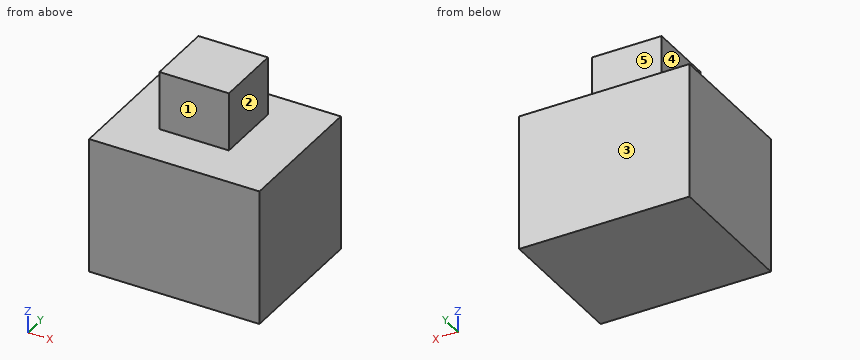
from build123d import *

# Parameters (mm, degrees)
F0_W     = 101.6
F0_H     = 105.0883368849
F1_DEPTH = 101.1590287089
F2_W     = 105.0883368849
F2_H     = 101.1590287089
F3_DEPTH = 25.4
F6_W     = 51.8510639668
F6_H     = 50.3680855036
F7_DEPTH = 43.5765609145


# Not quite as in the source:
# - the program builds the solid bodies; features that only make, move or delete a surface that nothing else refers to are left out


with BuildPart() as f1:
    # F0 (on Top) → F1 (new body)
    with BuildSketch(Plane.XY):
        with Locations((-2.9358975589, -0.3588087857)):
            Rectangle(F0_W, F0_H)
    extrude(amount=F1_DEPTH)

    # F2 (on face) → F3 (join)
    with BuildSketch(Plane.YZ.offset(47.8641024411)):
        with Locations((-0.3588087857, 50.5795143545)):
            Rectangle(F2_W, F2_H)
    extrude(amount=F3_DEPTH)

    # F6 (on face) → F7 (join)
    with BuildSketch(Plane.XY.offset(101.1590287089)):
        with Locations((5.4090619087, 5.453877151)):
            Rectangle(F6_W, F6_H)
    extrude(amount=F7_DEPTH)


solid = f1.part
Geometry: final body of the model. Coordinates: model frame, mm. Face numbers are marked on the shaded views. A direction names the side the tool comes from. Give positions to 0.01 mm unless a question says otherwise; leave off trailing zeros. Write each loop counter-clockwise with the first axis right and the second up, starting at its lowest first coordinate (ties: lowest second). Pieces come first, ordered by that corner, then holes. Notation, with made-up numbers: M 58,1.5 L 104,1.5 A33 cw 104,30.5 Z; hole C 17.5,36.25 d2. An arc over 180 degrees is marked long. Answer in a Markdown table with one row per item. Add a question column.
(1) Section A-A on x = 22. Return loops of the section in (y, z), and give its area (3 significant figures).
(2) Reachability of the marked faces 1, 2, 3, 4 and 5 from +Z, -Z, +X, -X, +Y, -Y: full face, straight path, thin tool, end or side. Return the list, or none.
(3) Section C-C on z = 112.5. Return loops of the section in (x, y), and give its area (3 significant figures).
(4) First-contact query: pin 1 (22 mm diameter, centred on y = 2, z = 119.5, fed in from -X); pin 2 (10 mm diameter, centred on x = -34, y = 11, fed in from +Z); pin 3 (22 mm diameter, centred on y = 5, z = 115, fed in from +X). Flat tips, straight axial feed; report the tip coordinate or a pass-through.
(5) Ray query, line 1 (Z direction, x = 12, y = 47); line 2 (Y direction, x = 7, z = 126); line 3 (X direction, y = -6, z = 130). Return the intervals inside material, ascending.
(6) Section D-D on y = 40. Return loops of the section in (x, z), and give its area (3 significant figures).
(7) Section B-B on y = 17.5. Return loops of the section in (x, z), and give its area (3 significant figures).
Result set:
| question | item | result |
|---|---|---|
| 1 | outline | M -52.9,0 L 52.19,0 L 52.19,101.16 L 30.64,101.16 L 30.64,144.74 L -19.73,144.74 L -19.73,101.16 L -52.9,101.16 Z |
| 1 | area | 12,800 mm^2 |
| 2 | face 1 | +Z, +X, -X, -Y |
| 2 | face 2 | +Z, +X, +Y, -Y |
| 2 | face 3 | +Z, -Z, +X, -X, +Y |
| 2 | face 4 | +Z, -X, +Y, -Y |
| 2 | face 5 | +Z, +X, -X, +Y |
| 3 | outline | M -20.52,-19.73 L 31.33,-19.73 L 31.33,30.64 L -20.52,30.64 Z |
| 3 | area | 2,610 mm^2 |
| 4 | pin 1 | stops at x = -20.52 |
| 4 | pin 2 | stops at z = 101.16 |
| 4 | pin 3 | stops at x = 31.33 |
| 5 | line 1 | z = 0 to 101.16 |
| 5 | line 2 | y = -19.73 to 30.64 |
| 5 | line 3 | x = -20.52 to 31.33 |
| 6 | outline | M -53.74,0 L 73.26,0 L 73.26,101.16 L -53.74,101.16 Z |
| 6 | area | 12,800 mm^2 |
| 7 | outline | M -53.74,0 L 73.26,0 L 73.26,101.16 L 31.33,101.16 L 31.33,144.74 L -20.52,144.74 L -20.52,101.16 L -53.74,101.16 Z |
| 7 | area | 15,100 mm^2 |
